from build123d import *

# Parameters (mm, degrees)
SKETCH1_R           = 16
BOSS_EXTRUDE1_DEPTH = 13
SKETCH2_R           = 7.5
BOSS_EXTRUDE2_DEPTH = 5
FILLET3_R           = 10
FILLET4_R           = 5
SKETCH3_R           = 2
BOSS_EXTRUDE3_DEPTH = 2


# Some blends are built 0.0001 mm under size
with BuildPart() as part:
    # Sketch1 → Boss-Extrude1 (new body)
    with BuildSketch(Plane(origin=(0, 0, 0), x_dir=(1, 0, 0), z_dir=(0, 1, 0))):
        with Locations(Location((0, 0, 0), (0, 0, 90))):
            Circle(SKETCH1_R)
    extrude(amount=BOSS_EXTRUDE1_DEPTH)

    # Sketch2 → Boss-Extrude2 (add)
    with BuildSketch(Plane(origin=(0, 13, 0), x_dir=(1, 0, 0), z_dir=(0, 1, 0))):
        with Locations(Location((0, 0, 0), (0, 0, 270))):
            Circle(SKETCH2_R)
    extrude(amount=BOSS_EXTRUDE2_DEPTH)

    # Fillet3
    # the kernel refuses this fillet: 10 mm, written as the material it takes off along each edge
    with BuildSketch(Plane(origin=(0, 13, 0), x_dir=(0, 0, -1), z_dir=(1, 0, 0))) as fillet3_piece_1:
        with BuildLine():
            CenterArc((6, -9.886859967), FILLET3_R, 0, 81.373073441)
            Line((7.5, 0), (7.53, 0.197737199))
            ThreePointArc((7.53, 0.197737199), (11.75, 0.2), (16, 0.2))
            Line((16, 0.2), (16.2, 0))
            Line((16.2, 0), (16.2, -9.886859967))
            Line((16.2, -9.886859967), (16, -9.886859967))
        make_face()
    revolve(axis=Axis((0, 13, 0), (0, 1, 0)), mode=Mode.SUBTRACT)

    # Fillet4
    fillet4_edges = [part.edges().sort_by_distance(p)[0] for p in [
        (0, 18, -7.5),
    ]]
    fillet(fillet4_edges, radius=FILLET4_R - 0.0001)  # a hair under: the kernel refuses the full size

    # Sketch3 → Boss-Extrude3 (add)
    with BuildSketch(Plane.XZ):
        with BuildLine():
            Line((6.757246285, 15.805857572), (23.195831847, 0.73715414))
            ThreePointArc((23.195831847, 0.73715414), (23.520107219, 0), (23.195831847, -0.73715414))
            Line((23.195831847, -0.73715414), (6.757246285, -15.805857572))
            ThreePointArc((6.757246285, -15.805857572), (0, -18.43431617), (-6.757246285, -15.805857572))
            Line((-6.757246285, -15.805857572), (-23.195831847, -0.73715414))
            ThreePointArc((-23.195831847, -0.73715414), (-23.520107219, 0), (-23.195831847, 0.73715414))
            Line((-23.195831847, 0.73715414), (-6.757246285, 15.805857572))
            ThreePointArc((-6.757246285, 15.805857572), (0, 18.43431617), (6.757246285, 15.805857572))
        make_face()
        with Locations(Location((20, 0, 0), (0, 0, 270))):
            Circle(SKETCH3_R, mode=Mode.SUBTRACT)
        with Locations(Location((-20, 0, 0), (0, 0, 90))):
            Circle(SKETCH3_R, mode=Mode.SUBTRACT)
    extrude(amount=BOSS_EXTRUDE3_DEPTH)


solid = part.part
Work out the finished part from the listing and answer in its coordinate system (mm). A direction names the side the tool comes from. Give positions to 0.01 mm unless a question says otherwise; leave off trailing zeros. Loops run counter-clockwise (first coordinate to the right, second up) from the corner with the lowest first, then second, coordinate; pieces in that order, holes last. Notation, with made-up numbers: (59, -14) - (74, -14) arc R13 ccw to (74, -4) - close; hole circle Ø3 at (52, -16). An arc over 180 degrees is marked (long way). Answer in a Markdown table with one row per item. Add a question column.
Q1. Each of these flat-tipped pins is pushed along its axis until it touches: P1, Ø5, axis at x = -20, z = 0, coming from the +Y side; P2, Ø12, axis at x = 10, z = -1.5, coming from the +Y side; P3, Ø6, axis at x = -12, y = 6.5, coming from the +Z side; P4, Ø3, axis at x = 20, z = 0, coming from the +Y side. Where does it stop, or does it pass through?
Q2. Determine the mould class of faces 1 (the cylindrical face through (22, -1, 0)), 2 (the cylindrical face through (15.62, 1.53, 3.47)), 3 (the flat face through (14.86, -0.99, 8.38)) for opening direction Z: released by +Z, released by -Z, zero draft, split by the parting line, or undercut.
Q3. A tool of negligible diameter and unlimited length cuts with its end or side. For faces 4 (the flat face through (-14.86, -0.99, -8.38)), 5 (the flat face through (-16, 0, -4)), from which of +Z, -Z, +X, -X, +Y, -Y can it reach the whole face along a straight path? Write none if from no direction.
Q4. The part is cut by section B-B (z = 0). State how many separate pieces and enclosed holes the cut face has, and give its area (3 significant figures).
Q5. Consider line 1 along Y through (x, z) = (-5, 17); line 2 along X through (y, z) = (0.25, -3); line 3 along Y through (x, z) = (4.5, 14.5). Determine where each line is inside the solid, lowest interval first.
Q6. The part is cut by section A-A (x = -20). Determine the outline of the cut face in (y, z).
Solution:
| question | item | result |
|---|---|---|
| 1 | P1 | stops at y = 0 |
| 1 | P2 | stops at y = 17.73 |
| 1 | P3 | stops at z = 12.76 |
| 1 | P4 | passes through |
| 2 | face 1 | undercut |
| 2 | face 2 | split by the parting line |
| 2 | face 3 | released by +Z |
| 3 | face 4 | -Z, -X, +Y, -Y |
| 3 | face 5 | +Y |
| 4 | separate pieces | 3 |
| 4 | enclosed holes | 0 |
| 4 | area | 517 mm² |
| 5 | line 1 | y = -2 to 0 |
| 5 | line 2 | x = -15.72 to 15.72 |
| 5 | line 3 | y = -2 to 7.07 |
| 6 | outline | (-2, -3.67) - (0, -3.67) - (0, -2) - (-2, -2) - close; (-2, 2) - (0, 2) - (0, 3.67) - (-2, 3.67) - close |
